Verification items for the finished model (mm, model axes). Give positions to 0.01 mm unless a question says otherwise; leave off trailing zeros. Write each loop counter-clockwise with the first axis right and the second up, starting at its lowest first coordinate (ties: lowest second). Pieces come first, ordered by that corner, then holes. Notation, with made-up numbers: (78.5, -20.75) - (85.5, -20.75) arc R10 cw to (85.5, -16.75) - close; hole circle Ø7 at (20.25, 56). An arc over 180 degrees is marked (long way). Answer as a JSON object with one key per item and string values. Group by question number.
Item 1: Go/stop test with a flat-tipped pin: pin 1 (6 mm diameter, centred on x = 0, z = 0, fed in from -Y). Record where the tip stops, or that it passes through.
Item 2: Sectioned sample at C-C, the plane z = 0. Record the boundary of the cut face in (x, y).
Item 3: Sectioned sample at D-D, the plane x = -31.75. Record the boundary of the cut face in (y, z), and give its area (3 significant figures).
Item 4: Sectioned sample at B-B, the plane y = 1.3. Record the boundary of the cut face in (x, z).
Item 5: Scan lines: line 1 along X through (y, z) = (1.3, 0); line 2 along Z through (x, y) = (-48, 1.45); line 3 along X through (y, z) = (1.9, -1.75). Record each from-to range of solid material in increasing order. Write a range as [from, to].
Item 6: Sectioned sample at A-A, the plane x = 0. Record the boundary of the cut face in (y, z), and give its area (3 significant figures).
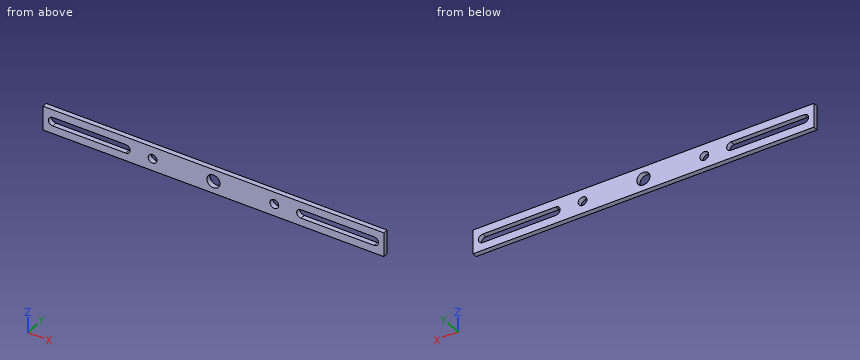
```python
from build123d import *

# Parameters (mm, degrees)
SKETCH1_W           = 177.8
SKETCH1_H           = 12.7
SKETCH1_R           = 3.429
SKETCH1_R_2         = 2.286
BOSS_EXTRUDE1_DEPTH = 2.54


with BuildPart() as part:
    # Sketch1 → Boss-Extrude1 (new body)
    with BuildSketch(Plane(origin=(0, 0, 0), x_dir=(1, 0, 0), z_dir=(0, 1, 0))):
        Rectangle(SKETCH1_W, SKETCH1_H)
        with Locations(Location((0, 0, 0), (0, 0, 270))):
            Circle(SKETCH1_R, mode=Mode.SUBTRACT)
        with Locations(Location((-31.75, 0, 0), (0, 0, 270))):
            Circle(SKETCH1_R_2, mode=Mode.SUBTRACT)
        with Locations(Location((31.75, 0, 0), (0, 0, 270))):
            Circle(SKETCH1_R_2, mode=Mode.SUBTRACT)
        with BuildLine():
            Line((-83.82, 2.286), (-45.72, 2.286))
            ThreePointArc((-45.72, 2.286), (-43.434, 0), (-45.72, -2.286))
            Line((-45.72, -2.286), (-83.82, -2.286))
            ThreePointArc((-83.82, -2.286), (-86.106, 0), (-83.82, 2.286))
        make_face(mode=Mode.SUBTRACT)
        with BuildLine():
            Line((83.82, -2.286), (45.72, -2.286))
            ThreePointArc((45.72, -2.286), (43.434, 0), (45.72, 2.286))
            Line((45.72, 2.286), (83.82, 2.286))
            ThreePointArc((83.82, 2.286), (86.106, 0), (83.82, -2.286))
        make_face(mode=Mode.SUBTRACT)
    extrude(amount=BOSS_EXTRUDE1_DEPTH)


solid = part.part
```
Geometry check:
{
 "1": {"pin 1": "through"},
 "2": {"outline": "(-88.9, 0) - (-86.11, 0) - (-86.11, 2.54) - (-88.9, 2.54) - close; (-43.43, 0) - (-34.04, 0) - (-34.04, 2.54) - (-43.43, 2.54) - close; (-29.46, 0) - (-3.43, 0) - (-3.43, 2.54) - (-29.46, 2.54) - close; (3.43, 0) - (29.46, 0) - (29.46, 2.54) - (3.43, 2.54) - close; (34.04, 0) - (43.43, 0) - (43.43, 2.54) - (34.04, 2.54) - close; (86.11, 0) - (88.9, 0) - (88.9, 2.54) - (86.11, 2.54) - close"},
 "3": {"outline": "(0, -6.35) - (2.54, -6.35) - (2.54, -2.29) - (0, -2.29) - close; (0, 2.29) - (2.54, 2.29) - (2.54, 6.35) - (0, 6.35) - close", "area": "20.6 mm^2"},
 "4": {"outline": "(-88.9, -6.35) - (88.9, -6.35) - (88.9, 6.35) - (-88.9, 6.35) - close; hole (-83.82, -2.29) - (-45.72, -2.29) arc R2.29 ccw to (-45.72, 2.29) - (-83.82, 2.29) arc R2.29 ccw to start; hole circle Ø4.57 at (-31.75, 0); hole circle Ø6.86 at (0, 0); hole circle Ø4.57 at (31.75, 0); hole (45.72, -2.29) - (83.82, -2.29) arc R2.29 ccw to (83.82, 2.29) - (45.72, 2.29) arc R2.29 ccw to start"},
 "5": {"line 1": "[-88.9, -86.11], [-43.43, -34.04], [-29.46, -3.43], [3.43, 29.46], [34.04, 43.43], [86.11, 88.9]", "line 2": "[-6.35, -2.29], [2.29, 6.35]", "line 3": "[-88.9, -85.29], [-44.25, -33.22], [-30.28, -2.95], [2.95, 30.28], [33.22, 44.25], [85.29, 88.9]"},
 "6": {"outline": "(0, -6.35) - (2.54, -6.35) - (2.54, -3.43) - (0, -3.43) - close; (0, 3.43) - (2.54, 3.43) - (2.54, 6.35) - (0, 6.35) - close", "area": "14.8 mm^2"}
}
